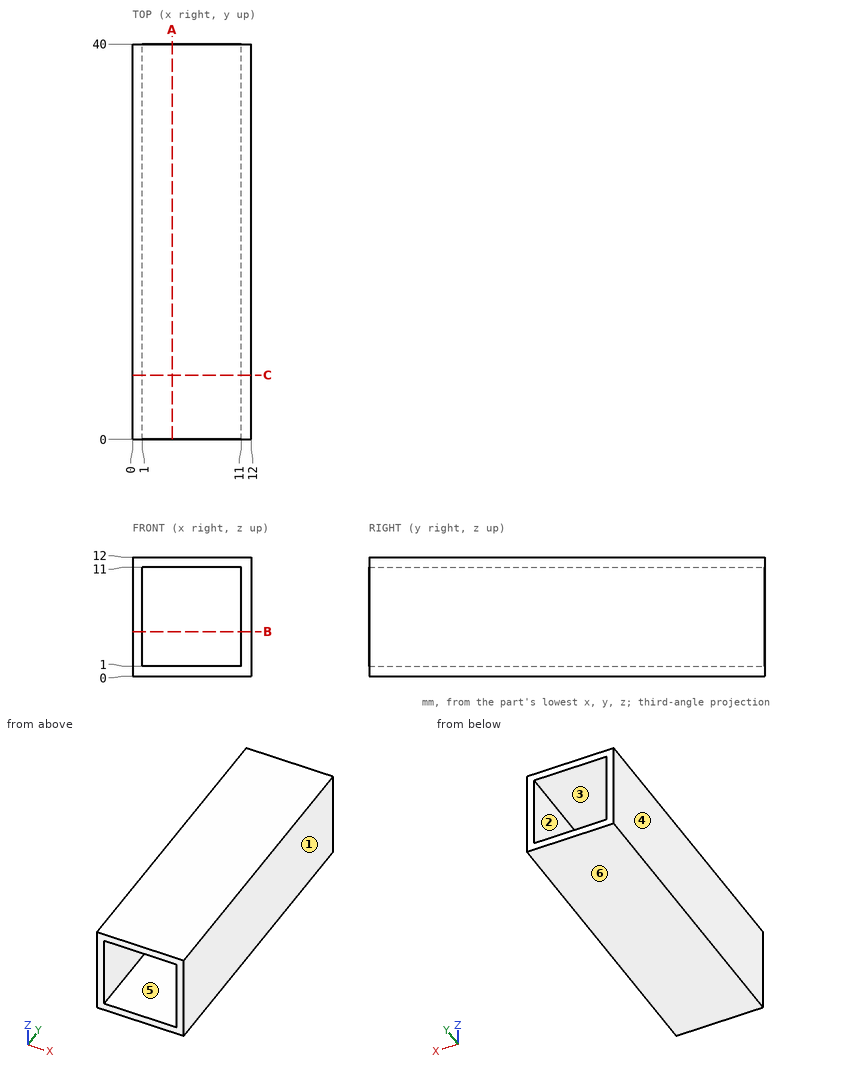
Design review of the part shown in the three views and the two pictorial views. Dimensions are in mm from the part's minimum x, y and z. A direction names the side the tool comes from. Coordinates: 2 decimals unless noted, no trailing zeros. Order: outer loops, then holes, each group sorted by start corner. A loop starts at its lowest first (then second) coordinate and runs counter-clockwise, first axis right, second up. Notation, with made-up numbers: (86.25, 4.25) -> (100.25, 4.25) arc R28 cw to (100.25, 40.25) -> close; hole circle Ø6 at (-2, 30.25). An arc over 180 degrees is marked (long way). Use one line per item in the form item = value. Start each with the question number.
(1) For probe 1 along Z at (x, y) = (9.5, 16), list the stretches that pass through material, from the lowest coordinate up.
(2) Add section C-C on y = 6.5. State the section outline as (x, z) points, plus the area to 3 significant figures.
(3) Add section A-A on x = 4. State the section outline as (y, z) points, plus the area to 3 significant figures.
(4) The part is to be moulded in two halves that separate along X. For the marked faces 3, 4, 5 and 6, say which applies: +X half, -X half, draft (parallel to the pull), parting line (faces both ways), or undercut.
(5) Add section B-B on z = 4.5. State the section outline as (x, y) points, plus the area to 3 significant figures.
(6) For the marked faces 1 and 2, list the 3-axis set-ups (+Z, -Z, +X, -X, +Y, -Y) from which the entire face can be reached by the end or side of a thin tool; tool diameter is ignored.
Answer block:
q1.probe_1 = 0 to 1, 11 to 12
q2.outline = (0, 0) -> (12, 0) -> (12, 12) -> (0, 12) -> close; hole (1, 1) -> (11, 1) -> (11, 11) -> (1, 11) -> close
q2.area = 44.0 mm²
q3.outline = (0, 0) -> (40, 0) -> (40, 1) -> (0, 1) -> close; (0, 11) -> (40, 11) -> (40, 12) -> (0, 12) -> close
q3.area = 80.0 mm²
q4.face_3 = undercut
q4.face_4 = -X half
q4.face_5 = undercut
q4.face_6 = draft
q5.outline = (0, 0) -> (1, 0) -> (1, 40) -> (0, 40) -> close; (11, 0) -> (12, 0) -> (12, 40) -> (11, 40) -> close
q5.area = 80.0 mm²
q6.face_1 = +Z, -Z, +X, +Y, -Y
q6.face_2 = +Y, -Y
